Solid Edge part; units mm, degrees
sketch "Sketch1" plane through (0, 0, 0) normal (0, -1, 0) x (1, 0, 0)
  line L0 (210, 0) -> (210, 105)
  line L1 (0, 0) -> (210, 0)
  line L2 (0, 105) -> (0, 0)
  arc A0 (0, 105) -> (210, 105) centre (105, 105) cw
extrude "Protrusion1" add sketch "Sketch1" against normal blind 30
sketch "Sketch2" plane through (0, 0, 0) normal (0, -1, 0) x (1, 0, 0)
  arc A0 (20, 105) -> (190, 105) centre (105, 105) cw
  line L0 (190, 105) -> (190, 20)
  line L1 (190, 20) -> (20, 20)
  line L2 (20, 20) -> (20, 105)
extrude "ExtrudedCutout_2" cut sketch "Sketch2" along normal mid plane 236.6242
sketch "Sketch3" plane through (0, 0, 0) normal (0, -1, 0) x (1, 0, 0)
  circle A0 centre (105.0544, 200.7425) radius 4
  line L0 (8.4015, 107.1927) -> (8.4015, 37.1927)
  line L1 (14.4015, 37.1927) -> (14.4015, 107.1927)
  arc A1 (14.4015, 37.1927) -> (8.4015, 37.1927) centre (11.4015, 37.1927) cw
  arc A2 (8.4015, 107.1927) -> (14.4015, 107.1927) centre (11.4015, 107.1927) cw
  line L2 (195.5985, 37.1927) -> (195.5985, 107.1927)
  arc A3 (201.5985, 107.1927) -> (195.5985, 107.1927) centre (198.5985, 107.1927) ccw
  line L3 (201.5985, 107.1927) -> (201.5985, 37.1927)
  arc A4 (195.5985, 37.1927) -> (201.5985, 37.1927) centre (198.5985, 37.1927) ccw
  line L4 (180.1885, 11.603) -> (30.1885, 11.603)
  line L5 (30.1885, 5.603) -> (180.1885, 5.603)
  arc A5 (30.1885, 5.603) -> (30.1885, 11.603) centre (30.1885, 8.603) cw
  arc A6 (180.1885, 11.603) -> (180.1885, 5.603) centre (180.1885, 8.603) cw
extrude "ExtrudedProtrusion_4" add sketch "Sketch3" along normal blind 5
Can you work these out from the model? Positions are in its coordinate system, mm. A direction names the side the tool comes from. Coordinates: 2 decimals unless noted, no trailing zeros. Loops run counter-clockwise (first coordinate to the right, second up) from the corner with the lowest first, then second, coordinate; pieces in that order, holes last. Notation, with made-up numbers: M 86,-24 L 144,-24 A22 cw 144,-18 Z; hole C 16.25,-3 d9. An arc over 180 degrees is marked long. Put each result on its own line as item: value. Start each with the question number.
(1) Imagine slicing it at B-B on x = 34. List the corners of the cut face in (y, z) for me, and give its area (3 significant figures).
(2) Will these pins go through, and if not, where does the flat tip stop? pin 1 Ø3 at (x, y) = (126.5, 22) entering from -Z; pin 2 Ø4 at (x, y) = (83.5, -3) entering from +Z; pin 3 Ø1.5 at (y, z) = (-2, 75.5) entering from +X; pin 4 Ø4 at (y, z) = (-2.5, 65.5) entering from -X.
(3) Imagine slicing it at D-D on x = 118. List the corners of the cut face in (y, z) for me.
(4) Imagine slicing it at C-C on z = 173. List the corners of the cut face in (x, y) for me, and give its area (3 significant figures).
(5) I need wall thicknesses on probe 1 along X at (y, z) = (22, 89.5); probe 2 along X at (y, z) = (-1, 64); probe 3 along Y at (x, z) = (8, 57). Which ranges of each line are inside material? Lowest first, please.
(6) Imagine slicing it at A-A on y = 12. List the corners of the cut face in (x, z) for me.
(7) Which directions (+Z, -Z, +X, -X, +Y, -Y) give clear straight access to the entire face, cutting with the end or side of a thin tool? Please do faces 1 (the face through (105, 0, 12)), 2 (the face through (201.598, -2, 73)), 3 (the face through (27.19, -2.46, 8.54)), 4 (the face through (103.13, 15.21, 189.98)).
(8) We'd pull the mould along X, two halves only. Please class faces 5 (the face through (195.598, -2, 72)), 6 (the face through (104.534, -2.465, 196.777)), 7 (the face through (106, -2, 11.603)): +X half, -X half, draft (parallel to the pull), parting line (faces both ways), or undercut.
Worked answers:
1. outline: M -5,5.6 L 0,5.6 L 0,0 L 30,0 L 30,20 L 0,20 L 0,11.6 L -5,11.6 Z; M 0,151.73 L 30,151.73 L 30,182.36 L 0,182.36 Z
1. area: 1,550 mm2
2. pin 1: stops at z = 0
2. pin 2: stops at z = 11.6
2. pin 3: stops at x = 201.6
2. pin 4: stops at x = 8.4
3. outline: M -5,5.6 L 0,5.6 L 0,0 L 30,0 L 30,20 L 0,20 L 0,11.6 L -5,11.6 Z; M 0,189 L 30,189 L 30,209.19 L 0,209.19 Z
4. outline: M 24.99,0 L 54,0 L 54,30 L 24.99,30 Z; M 156,0 L 185.01,0 L 185.01,30 L 156,30 Z
4. area: 1,740 mm2
5. probe 1: x = 0 to 20, 190 to 210
5. probe 2: x = 8.4 to 14.4, 195.6 to 201.6
5. probe 3: y = 0 to 30
6. outline: M 0,0 L 210,0 L 210,105 A105 ccw 0,105 Z; hole M 20,20 L 190,20 L 190,105 A85 ccw 20,105 Z
7. face 1: -Y
7. face 2: +Z, -Z, +X, -Y
7. face 3: -X, -Y
7. face 4: +Y, -Y
8. face 5: undercut
8. face 6: parting line
8. face 7: draft
